Design review of the part built by this model. Coordinates are the model's own, in mm. Coordinates: 2 decimals unless noted, no trailing zeros. Order: outer loops, then holes, each group sorted by start corner. A loop starts at its lowest first (then second) coordinate and runs counter-clockwise, first axis right, second up. Notation, with made-up numbers: M -40,17 L 13,17 A17 cw 13,34 Z; hole C -11.75,53.5 d7. An arc over 180 degrees is marked long. Answer as a JSON object with one key per item and string values.
Autodesk Inventor part; units mm, degrees
ref_plane "YZ Plane" through (0, 0, 0) normal (1, 0, 0) x (0, 1, 0)
ref_plane "XZ Plane" through (0, 0, 0) normal (0, 1, 0) x (-1, 0, 0)
ref_plane "XY Plane" through (0, 0, 0) normal (0, 0, 1) x (1, 0, 0)
ref_plane "Work Plane1" through (-244.516826, 0, -292.10783) normal (0, -1, 0) x (1, 0, 0)
sketch "Sketch1" plane through (-244.516826, 0, -292.10783) normal (0, -1, 0) x (1, 0, 0)
  line L0 (-82.234926, -443.016385) -> (-82.234926, 4.14342)
  line L1 (16.056549, -523.499895) -> (-89.634926, -493.408338)
  line L2 (-82.234926, 4.14342) -> (116.599095, 288.10783)
  line L3 (116.599095, 288.10783) -> (240.516826, 288.10783)
  line L4 (590.833218, -28.092085) -> (443.497514, 287.870352)
  line L5 (590.833218, -526.137374) -> (590.833218, -28.092085)
  point P0 (244.516826, 292.10783)
sketch "Sketch2" plane through (-244.516826, 0, -292.10783) normal (0, -1, 0) x (1, 0, 0)
  line L0 (16.056549, -523.499895) -> (-82.234926, -495.466532)
  line L1 (-82.234926, -495.466532) -> (-82.234926, 4.14342)
  line L2 (-82.234926, 4.14342) -> (116.599095, 288.10783)
  line L3 (116.599095, 288.10783) -> (443.497514, 287.870352)
  line L4 (443.497514, 287.870352) -> (590.833218, -28.092085)
  line L5 (590.833218, -28.092085) -> (590.833218, -526.137374)
  line L6 (590.833218, -523.499895) -> (16.056549, -523.499895)
  point P0 (244.516826, 292.10783)
sketch "Sketch2 outline for Plate extrude" plane through (-244.516826, 0, -292.10783) normal (0, -1, 0) x (1, 0, 0)
  line L0 (16.056549, -523.499895) -> (-82.234926, -495.466532)
  line L1 (-82.234926, -495.466532) -> (-82.234926, 4.14342)
  line L2 (-82.234926, 4.14342) -> (116.599095, 288.10783)
  line L3 (116.599095, 288.10783) -> (443.497514, 287.870352)
  line L4 (443.497514, 287.870352) -> (590.833218, -28.092085)
  line L5 (590.833218, -28.092085) -> (590.833218, -526.137374)
  line L6 (590.833218, -526.137374) -> (16.056549, -523.499895)
extrude "Plate extrude" add sketch "Sketch2 outline for Plate extrude" against normal blind 1.6
sketch "Sketch3" plane through (-244.516826, 0, -292.10783) normal (0, -1, 0) x (1, 0, 0)
  circle A0 centre (303.423661, -47.967523) radius 80.5 construction
  circle A1 centre (303.423661, -45.120279) radius 75 construction
  line L0 (153.423661, 104.879721) -> (453.423661, 104.879721)
  line L1 (453.423661, 104.879721) -> (453.423661, -195.120279)
  line L2 (453.423661, -195.120279) -> (153.423661, -195.120279)
  line L3 (153.423661, -195.120279) -> (153.423661, 104.879721)
  line L4 (153.423661, 104.879721) -> (453.423661, -195.120279) construction
  line L5 (453.423661, 104.879721) -> (153.423661, -195.120279) construction
  point P0 (244.516826, 292.10783)
  dimension "d3" = 300
  dimension "d4" = 300
extrude "Tailstock door" [suppressed]
sketch "Sketch4" plane through (-244.516826, 0, -292.10783) normal (0, -1, 0) x (1, 0, 0)
  circle A0 centre (303.423661, -45.120279) radius 75 construction
  circle A1 centre (303.423661, -45.120279) radius 81.28
  circle A2 centre (303.423661, -45.330045) radius 80.5 construction
  point P0 (244.516826, 292.10783)
  dimension "d7" = 162.56
  dimension "d8" = 161
extrude "Headstock cut out" [suppressed]
sketch "Sketch5" plane through (-244.516826, 1.6, -292.10783) normal (0, 1, 0) x (1, 0, 0)
  point P0 (244.516826, -292.10783)
  point P1 (303.423661, 45.330045)
properties part number "side cover plate.ipt-01"
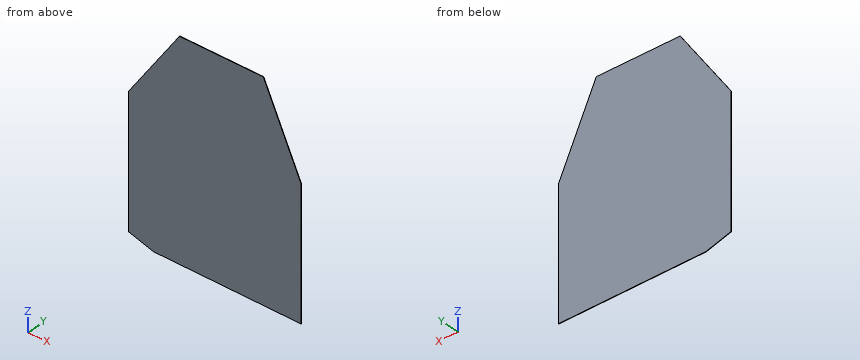
1) Add section C-C (z = -229). State the section outline as (x, y) points.
Taken from the geometry:
{"outline": "M -285.46,0 L 303.79,0 L 303.79,1.6 L -285.46,1.6 Z"}
2) Add section B-B (x = -250.5). State the section outline as (y, z) points.
Taken from the geometry:
{"outline": "M 0,-809.32 L 1.6,-809.32 L 1.6,-179.07 L 0,-179.07 Z"}
3) Add section A-A (y = 0.95). State the section outline as (x, z) points, and give its area (3 significant figures).
Taken from the geometry:
{"outline": "M -326.75,-787.57 L -228.46,-815.61 L 346.32,-818.25 L 346.32,-320.2 L 198.98,-4.24 L -127.92,-4 L -326.75,-287.96 Z", "area": "494,000 mm2"}
4) To check wall thickness, follow L1, parallel to Z at x = 264, y = 1.3; L2, parallel to X at y = 0.5, z = -88; L3, parallel to Z at x = 145, y = 1.4. State the ranges of each line that lie inside material, in increasing order.
Taken from the geometry:
{"L1": "z = -817.87 to -143.67", "L2": "x = -186.74 to 238.04", "L3": "z = -817.32 to -4.2"}
